```python
from build123d import *

# Parameters (mm, degrees)
F1_DEPTH  = 51.054
F2_R      = 6.34999
F3_W      = 41.275
F3_H      = 19.05
F4_DEPTH  = 76.2
F5_SIZE2  = 3.302
F5_SIZE   = 3.302
F6_W      = 44.45
F6_H      = 19.05
F7_DEPTH  = 3.175
F8_R      = 4.826
F9_DEPTH  = 16.002
F10_R     = 4.7625
F11_DEPTH = 12.7
F12_W     = 66.675
F12_H     = 19.05
F13_DEPTH = 9.525
F15_DEPTH = 76.2
F16_W     = 67.945
F16_H     = 19.05
F17_DEPTH = 9.525
F19_DEPTH = 85.4085


# Not quite as in the source:
# - a fillet or chamfer is up to 0.001 mm smaller than in the source, because OpenCascade refuses the exact size


with BuildPart() as f1:
    # F0 (on Front) → F1 (new body)
    with BuildSketch(Plane.XZ):
        Polygon((-38.7827743664, 8.7870896519), (-16.9203323245, 8.7870896519), (-16.9203323245, -16.6129103481), (59.6422256336, -16.6129103481), (59.6422256336, 21.4870896519), (5.6545256336, 21.4870896519), (5.6545256336, 27.8370896519), (-15.0464743664, 27.8370896519), (-15.0464743664, 21.4870896519), (-21.3202743664, 21.4870896519), (-21.3202743664, 27.8370896519), (-38.7827743664, 27.8370896519), align=None)
    extrude(amount=F1_DEPTH)

    # F2 (radius 6.35 in the source; OpenCascade refuses exactly that, so slightly less here)
    f2_edges = [f1.edges().sort_by_distance(p)[0] for p in [
        (5.654526, -25.527, 21.48709),
    ]]
    fillet(f2_edges, radius=F2_R)

    # F3 (on face) → F4 (cut)
    with BuildSketch(Plane.XY.offset(21.4870896519)):
        with Locations((39.0047256336, -25.527)):
            Rectangle(F3_W, F3_H)
    extrude(amount=-F4_DEPTH, mode=Mode.SUBTRACT)

    # F5
    f5_edges = [f1.edges().sort_by_distance(p)[0] for p in [
        (59.642226, -51.054, 2.43709),
        (59.642226, 0, 2.43709),
    ]]
    chamfer(f5_edges, length=F5_SIZE, length2=F5_SIZE2)

    # F6 (on face) → F7 (cut)
    with BuildSketch(Plane.XY.offset(27.8370896519)):
        with Locations((-16.5577743664, -36.7665)):
            Rectangle(F6_W, F6_H)
    extrude(amount=-F7_DEPTH, mode=Mode.SUBTRACT)

    # F8 (on face) → F9 (cut)
    with BuildSketch(Plane.YZ.offset(59.6422256336)):
        with Locations((-42.9895, 2.4370896519)):
            Circle(F8_R)
        with Locations((-8.0645, 2.4370896519)):
            Circle(F8_R)
    extrude(amount=-F9_DEPTH, mode=Mode.SUBTRACT)

    # F10 (on face) → F11 (cut)
    with BuildSketch(Plane.XY.offset(27.8370896519)):
        with Locations((-29.8927743664, -19.05)):
            Circle(F10_R)
        with Locations((-4.4927743664, -19.05)):
            Circle(F10_R)
    extrude(amount=-F11_DEPTH, mode=Mode.SUBTRACT)

    # F12 (on face) → F13 (join)
    with BuildSketch(Plane.XZ.offset(51.054)):
        with Locations((12.0172256336, 0.9130896519)):
            Rectangle(F12_W, F12_H)
    extrude(amount=F13_DEPTH)

    # F14 (on face) → F15 (cut)
    with BuildSketch(Plane.YZ.offset(45.3547256336)):
        Polygon((-60.579, -6.2306603481), (-51.054, 10.4380896519), (-60.579, 10.4380896519), align=None)
    extrude(amount=-F15_DEPTH, mode=Mode.SUBTRACT)

    # F16 (on face) → F17 (join)
    with BuildSketch(Plane(origin=(0, 0, 0), x_dir=(-1, 0, 0), z_dir=(0, 1, 0))):
        with Locations((-12.6522256336, 0.9130896519)):
            Rectangle(F16_W, F16_H)
    extrude(amount=F17_DEPTH)

    # F18 (on face) → F19 (cut, through all)
    with BuildSketch(Plane.YZ.offset(46.6247256336)):
        Polygon((0, 10.4380896519), (9.525, -6.2306603481), (9.525, 10.4380896519), align=None)
    extrude(amount=-F19_DEPTH, mode=Mode.SUBTRACT)


solid = f1.part
```
Can you work these out from the model? Positions are in its coordinate system, mm. A direction names the side the tool comes from. Give positions to 0.01 mm unless a question says otherwise; leave off trailing zeros. Order: outer loops, then holes, each group sorted by start corner. A loop starts at its lowest first (then second) coordinate and runs counter-clockwise, first axis right, second up. Notation, with made-up numbers: (31.25, -16) - (63.25, -16) arc R21 ccw to (63.25, -9) - close; hole circle Ø3 at (22.5, 56.5). An arc over 180 degrees is marked (long way). Use a Markdown table: item, result. Add a question column.
Q1. Please list where these lines run through material, in increasing order: line 1 along X through (y, z) = (-19, 19); line 2 along Y through (x, z) = (-7, 25.5); line 3 along Y through (x, z) = (32, 20.5).
Q2. If we section it at D-D on y = -29.5: Write out the boundary of the cut face in (x, z).
Q3. If we mould it in two halves opening along X, with no side actions, what happens to faces 4 (the flat face through (-30, -13, 27.837)), 5 (the flat face through (-21.32, -55, -1)), 6 (the flat face through (-18, -25, 21.487)), 7 (the cylindrical face through (0.05, -17.62, 21.58))? For each: released by +X, released by -X, zero draft, split by the parting line, or undercut.
Q4. On a 3-axis mill with a long thin cutter (end or side, diameter ignored), from which of +Z, -Z, +X, -X, +Y, -Y can I reach the whole of each face in a straight line? I mean faces 1 (the flat face through (-30, -37, 24.662)), 2 (the cylindrical face through (51.75, -47.81, 2.65)), 3 (the flat face through (39, -35.052, 3)). Say none if no direction works.
Q5. If we section it at B-B on z = 20: Count the separate pieces of the cut face and the enclosed holes in it, plus the area to 3 significant figures.
Q6. If we section it at A-A on x = 50: Write out the boundary of the cut face in (y, z).
Q7. If we section it at C-C on x = 35.5: Write out the boundary of the cut face in (y, z) (3 decimals).
Q8. I'm going to push flat-ended pins straight in: pin 1 (7.5 mm diameter, centred on y = -45, z = 2.5, fed in from +X); pin 2 (3 mm diameter, centred on y = -57, z = 0, fed in from -X); pin 3 (1.5 mm diameter, centred on x = 32.5, y = -53.5, fed in from -Z); pin 4 (1.5 mm diameter, centred on x = 49, z = 2.5, fed in from +Y). Where does each tip first touch, or does it pass through?
Answers follow:
| question | item | result |
|---|---|---|
| 1 | line 1 | x = -38.78 to -34.66, -25.13 to -9.26, 0.27 to 18.37 |
| 1 | line 2 | y = -51.05 to -46.29, -27.24 to -23.1, -15 to 0 |
| 1 | line 3 | y = -51.05 to -35.05, -16 to 0 |
| 2 | outline | (-38.78, 8.79) - (-16.92, 8.79) - (-16.92, -16.61) - (18.37, -16.61) - (18.37, 21.49) - (12, 21.49) arc R6.35 cw to (5.67, 27.44) - (5.67, 24.66) - (-15.05, 24.66) - (-15.05, 21.49) - (-21.32, 21.49) - (-21.32, 24.66) - (-38.78, 24.66) - close |
| 3 | face 4 | zero draft |
| 3 | face 5 | released by -X |
| 3 | face 6 | undercut |
| 3 | face 7 | undercut |
| 4 | face 1 | +Z, -X |
| 4 | face 2 | +X |
| 4 | face 3 | +Z, -Z, +X |
| 5 | separate pieces | 1 |
| 5 | enclosed holes | 2 |
| 5 | area | 4,090 mm^2 |
| 6 | outline | (-51.05, -16.61) - (-35.05, -16.61) - (-35.05, 21.49) - (-51.05, 21.49) - close; (-16, -16.61) - (0, -16.61) - (0, 21.49) - (-16, 21.49) - close; hole circle Ø9.65 at (-42.99, 2.44); hole circle Ø9.65 at (-8.06, 2.44) |
| 7 | outline | (-60.579, -8.612) - (-51.054, -8.612) - (-51.054, -16.613) - (-35.052, -16.613) - (-35.052, 21.487) - (-51.054, 21.487) - (-51.054, 10.438) - (-60.579, -6.231) - close; (-16.002, -16.613) - (0, -16.613) - (0, -8.612) - (9.525, -8.612) - (9.525, -6.231) - (0, 10.438) - (0, 21.487) - (-16.002, 21.487) - close |
| 8 | pin 1 | stops at x = 59.64 |
| 8 | pin 2 | stops at x = -21.32 |
| 8 | pin 3 | stops at z = -8.61 |
| 8 | pin 4 | stops at y = 0 |
